Input: dimensioned drawing with shaded views. Units: mm. Origin: part minimum x, y, z. Round coordinates to 2 decimals unless told otherwise and drop trailing zeros. Order: outer loops, then holes, each group sorted by start corner. A loop starts at its lowest first (then second) coordinate and runs counter-clockwise, first axis right, second up. Notation, with made-up numbers: M -3.5,10 L 10.5,10 A18 ccw 10.5,31 Z; hole C 52.5,59 d2. An arc over 180 degrees is marked long. Use one line per item in the form item = value. Start each with the question number.
Q1. Material intervals for probe 1 along Z at (x, y) = (38.1, 39.5) (3 decimals); probe 2 along X at (y, z) = (22, 27); probe 3 along Z at (x, y) = (22.5, 46.5), sorted ascending.
Q2. Pull-direction query (Z, two-part tool) for the marked faces 1, 2 and 3; classes: pulls with the +Z half, pulls with the -Z half, needs draft (parallel to the pull), parting line crosses it, or undercut.
Q3. Section B-B (z = 25.4). Return the cut outline in (x, y) (3 decimals).
Q4. Section C-C (y = 28). Return the cut outline in (x, z) (3 decimals), plus the area to 3 significant figures.
Q5. Section A-A (x = 25.4). Return the cut outline in (y, z) (3 decimals).
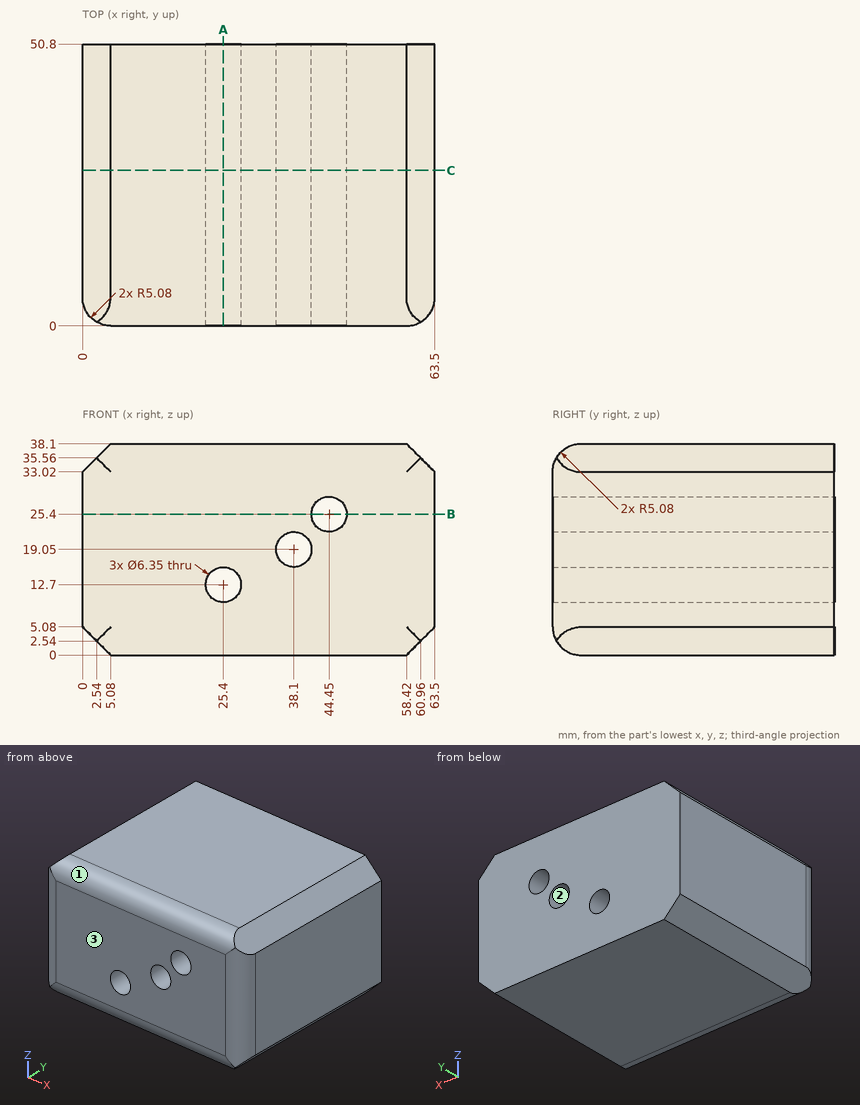
Results list:
q1.probe_1 = 0 to 15.875, 22.225 to 38.1
q1.probe_2 = 0 to 41.71, 47.19 to 63.5
q1.probe_3 = 0 to 11.41, 13.99 to 38.1
q2.face_1 = pulls with the +Z half
q2.face_2 = undercut
q2.face_3 = needs draft
q3.outline = M 0,5.08 A5.08 ccw 5.08,0 L 41.275,0 L 41.275,50.8 L 0,50.8 Z; M 47.625,0 L 58.42,0 A5.08 ccw 63.5,5.08 L 63.5,50.8 L 47.625,50.8 Z
q4.outline = M 0,5.08 L 5.08,0 L 58.42,0 L 63.5,5.08 L 63.5,33.02 L 58.42,38.1 L 5.08,38.1 L 0,33.02 Z; hole C 25.4,12.7 d6.35; hole C 38.1,19.05 d6.35; hole C 44.45,25.4 d6.35
q4.area = 2,270 mm2
q5.outline = M 0,5.08 A5.08 ccw 5.08,0 L 50.8,0 L 50.8,9.525 L 0,9.525 Z; M 0,15.875 L 50.8,15.875 L 50.8,38.1 L 5.08,38.1 A5.08 ccw 0,33.02 Z
